Verification items for the finished model (mm, model axes). Face numbers are marked on the shaded views. A direction names the side the tool comes from. Coordinates: 2 decimals unless noted, no trailing zeros. Order: outer loops, then holes, each group sorted by start corner. A loop starts at its lowest first (then second) coordinate and runs counter-clockwise, first axis right, second up. Notation, with made-up numbers: M 28,-9.75 L 49,-9.75 A12 cw 49,-0.75 Z; hole C -36,70.5 d3. An arc over 180 degrees is marked long. Return JSON: item names as keys, results as strings. Group by question number.
1. Section check C-C, the plane z = 4. Record the cut outline in (x, y), plus the area to 3 significant figures.
2. Section check B-B, the plane x = 0. Record the cut outline in (y, z), plus the area to 3 significant figures.
3. Material ranges on line 1 along Y through (x, z) = (-7, 19); line 2 along Y through (x, z) = (-3.5, -5.5); line 3 along Z through (x, y) = (0, 9.15), recorded low to high.
4. Gauge pin test, flat ends, axial feed: pin 1 (4 mm diameter, centred on x = 0, z = 0, fed in from +Y); pin 2 (2 mm diameter, centred on x = -1.5, y = 7, fed in from -Z); pin 3 (4.5 mm diameter, centred on x = 0, z = 0, fed in from -Y). Record the tip position at first contact, or that the pin passes through.
5. Mould release check, pull along X, two halves, no side actions. Record for the marked faces 4, 5, 6 and 7: +X half, -X half, draft (parallel to the pull), parting line (faces both ways), or undercut.
6. Section check A-A, the plane y = 8.5. Record the cut outline in (x, z), plus the area to 3 significant figures.
7. Set-up check for the marked faces 1, 2 and 3: record each of +Z, -Z, +X, -X, +Y, -Y from which the full face is reachable in a straight line by a thin tool's end or side.
8. Section check D-D, the plane z = 16. Record the cut outline in (x, y), plus the area to 3 significant figures.
```python
from build123d import *

# Parameters (mm, degrees)
SKETCH264_R           = 2.2
PAD066_DEPTH          = 10
POCKET176_DEPTH       = 10.001
POCKET176_DEPTH_BACK  = 10.001
SKETCH265_W           = 15.5
SKETCH265_H           = 15.5
POCKET177_DEPTH       = 23.501
CYLINDER014_R         = 0.5
CYLINDER014_DEPTH     = 20
CYLINDER015_R         = 0.5
CYLINDER015_DEPTH     = 20
POLARPATTERN005_COUNT = 4
SKETCH271_R           = 2.8
POCKET189_DEPTH       = 4
CHAMFER_SIZE          = 0.4


with BuildPart() as part:
    # Sketch264 → Pad066 (new body, symmetric)
    with BuildSketch(Plane.XZ):
        with BuildLine():
            ThreePointArc((-10, -4.2e-05), (2.1e-05, -10), (10, 0))
            Line((10, 0), (10, 11.5))
            Line((10, 12), (10, 11.5))
            Line((10, 36.5), (10, 12))
            Line((-10, 36.5), (10, 36.5))
            Line((-10, 12), (-10, 36.5))
            Line((-10, 11.5), (-10, 12))
            Line((-10, -4.2e-05), (-10, 11.5))
        make_face()
        Circle(SKETCH264_R, mode=Mode.SUBTRACT)
    extrude(amount=PAD066_DEPTH, both=True)

    # Sketch263 → Pocket176 (cut, two sides)
    with BuildSketch(Plane.YZ) as pocket176_sk:
        Polygon((-6, 11.5), (-6, -11), (-10, -11), (-10, 11.5), (-11.5, 13), (-11.5, -13), (11.5, -13), (11.5, 13), (10, 11.5), (10, -11), (6, -11), (6, 11.5), align=None)
    extrude(amount=-POCKET176_DEPTH, mode=Mode.SUBTRACT)
    extrude(pocket176_sk.sketch, amount=POCKET176_DEPTH_BACK, mode=Mode.SUBTRACT)

    # Sketch265 → Pocket177 (cut, through all)
    with BuildSketch(Plane.XY.offset(13)):
        Rectangle(SKETCH265_W, SKETCH265_H)
    extrude(amount=POCKET177_DEPTH, mode=Mode.SUBTRACT)

    # Cylinder014 → Cylinder014 (join)
    with BuildSketch(Plane(origin=(7.75, -2.5, 15), x_dir=(1, 0, 0), z_dir=(0, 0, 1))):
        Circle(CYLINDER014_R)
    cylinder014 = extrude(amount=CYLINDER014_DEPTH)

    # Cylinder015 → Cylinder015 (join)
    with BuildSketch(Plane(origin=(7.75, 2.5, 15), x_dir=(1, 0, 0), z_dir=(0, 0, 1))):
        Circle(CYLINDER015_R)
    cylinder015 = extrude(amount=CYLINDER015_DEPTH)

    # PolarPattern005: Cylinder014, Cylinder015 ×4 about axis
    polarpattern005_axis = Axis((0, 0, 0), (0, 0, 1))
    for i in range(1, POLARPATTERN005_COUNT):
        add(cylinder014.rotate(polarpattern005_axis, i * 360 / POLARPATTERN005_COUNT))
        add(cylinder015.rotate(polarpattern005_axis, i * 360 / POLARPATTERN005_COUNT))

    # Sketch271 → Pocket189 (cut)
    with BuildSketch(Plane.XZ.offset(10)):
        Circle(SKETCH271_R)
    extrude(amount=-POCKET189_DEPTH, mode=Mode.SUBTRACT)

    # Chamfer
    chamfer_edges = [part.edges().sort_by_distance(p)[0] for p in [
        (10, 0, 36.5),
        (0, -10, 36.5),
        (-10, 0, 36.5),
        (0, 10, 36.5),
    ]]
    chamfer(chamfer_edges, length=CHAMFER_SIZE)


solid = part.part
```
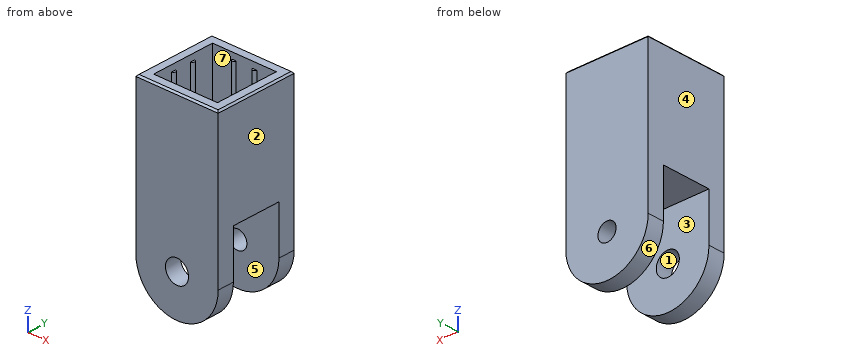
Answers follow:
{
 "1": {"outline": "M -10,-10 L 10,-10 L 10,-6 L -10,-6 Z; M -10,6 L 10,6 L 10,10 L -10,10 Z", "area": "160 mm^2"},
 "2": {"outline": "M -10,-10 L -6,-10 L -6,-2.8 L -10,-2.8 Z; M -10,2.8 L -6,2.8 L -6,11.5 L 6,11.5 L 6,2.2 L 10,2.2 L 10,36.1 L 9.6,36.5 L 7.75,36.5 L 7.75,13 L -7.75,13 L -7.75,36.5 L -9.6,36.5 L -10,36.1 Z; M 6,-10 L 10,-10 L 10,-2.2 L 6,-2.2 Z", "area": "268 mm^2"},
 "3": {"line 1": "-10 to -7.75, 7.75 to 10", "line 2": "-10 to -6, 6 to 10", "line 3": "-10 to -2.2, 2.2 to 36.5"},
 "4": {"pin 1": "through", "pin 2": "z = -9.99", "pin 3": "y = 6"},
 "5": {"face 4": "-X half", "face 5": "draft", "face 6": "parting line", "face 7": "undercut"},
 "6": {"outline": "M -10,0 A10 ccw 10,0 L 10,36.1 L 9.6,36.5 L -9.6,36.5 L -10,36.1 Z; hole C 0,0 d4.4", "area": "872 mm^2"},
 "7": {"face 1": "-Y", "face 2": "+Z, -Z, +X, +Y, -Y", "face 3": "-Z, +X, -X"},
 "8": {"outline": "M -10,-10 L 10,-10 L 10,10 L -10,10 Z; hole M -7.75,-7.75 L -3,-7.75 A0.5 cw -2,-7.75 L 2,-7.75 A0.5 cw 3,-7.75 L 7.75,-7.75 L 7.75,-3 A0.5 cw 7.75,-2 L 7.75,2 A0.5 cw 7.75,3 L 7.75,7.75 L 3,7.75 A0.5 cw 2,7.75 L -2,7.75 A0.5 cw -3,7.75 L -7.75,7.75 L -7.75,3 A0.5 cw -7.75,2 L -7.75,-2 A0.5 cw -7.75,-3 Z", "area": "163 mm^2"}
}
